from build123d import *

# Parameters (mm, degrees)
SKETCH1_R                      = 4.1275
BOSS_EXTRUDE1_DEPTH            = 22.225
F_7_0_201_DIAMETER_HOLE1_D     = 5.1054
F_7_0_201_DIAMETER_HOLE1_DEPTH = 1.27
F_10_32_TAPPED_HOLE1_D         = 4.0386


with BuildPart() as part:
    # Sketch1 → Boss-Extrude1 (new body)
    with BuildSketch(Plane.XY):
        Circle(SKETCH1_R)
    extrude(amount=BOSS_EXTRUDE1_DEPTH)

    # #7 (0.201) Diameter Hole1
    with Locations(Plane(origin=(0, 4.1275, 9.525), x_dir=(1, 0, 0), z_dir=(0, 1, 0))):
        with Locations((0, 0)):
            Hole(F_7_0_201_DIAMETER_HOLE1_D / 2, depth=F_7_0_201_DIAMETER_HOLE1_DEPTH)

    # #10-32 Tapped Hole1 (through all)
    with Locations(Plane(origin=(0, 4.1275, 9.525), x_dir=(1, 0, 0), z_dir=(0, 1, 0))):
        with Locations((0, 0)):
            Hole(F_10_32_TAPPED_HOLE1_D / 2)


solid = part.part
Part model, mm, in its own coordinate system. Give positions to 0.01 mm unless a question says otherwise; leave off trailing zeros. Loops run counter-clockwise (first coordinate to the right, second up) from the corner with the lowest first, then second, coordinate; pieces in that order, holes last.
(1) Band-saw the part on D-D (y = -1). Write the cut outline in (x, z) (3 decimals).
Return value:
outline: (-4.005, 0) - (4.005, 0) - (4.005, 22.225) - (-4.005, 22.225) - close; hole circle Ø4.039 at (0, 9.525)
(2) Pull direction X, two halves, no side cores. Call faces 1 (the cylindrical face through (2.026, 3.345, 11.078)), 2 (the flat face through (0, 0, 0)), 3 (the cylindrical face through (1.905, -3.662, 10.957)), 4 (the cylindrical face through (2.017, -0.686, 9.436)): pulls with the +X half, pulls with the -X half, needs draft (parallel to the pull), parting line crosses it, or undercut.
Return value:
face 1: undercut
face 2: needs draft
face 3: parting line crosses it
face 4: undercut
(3) Drill centre lines: line 1 along Z through (x, y) = (0, 3.65) (3 decimals); line 2 along Z through (x, y) = (-1, -3) (3 decimals); line 3 along Y through (x, z) = (-2.5, 18). Where is each one in solid material? Low to high.
Return value:
line 1: z = 0 to 6.972, 12.078 to 22.225
line 2: z = 0 to 7.771, 11.279 to 22.225
line 3: y = -3.28 to 3.28
(4) Pin check, flat tip, straight feed: pin 1 (2 mm diameter, centred on y = 2, z = 14, fed in from -X). Stop position of the tip, or through.
Return value:
pin 1: stops at x = -4
(5) Band-saw the part on C-C (y = 3.5). Write the cut outline in (x, z) (3 decimals), and give its area (3 significant figures).
Return value:
outline: (-2.188, 0) - (2.188, 0) - (2.188, 8.21) arc R2.553 cw to (-2.188, 8.21) - close; (-2.188, 10.84) arc R2.553 cw to (2.188, 10.84) - (2.188, 22.225) - (-2.188, 22.225) - close
area: 78.1 mm2
(6) Band-saw the part on A-A (x = 0). Write the cut outline in (y, z) (1 decimal), and give its area (3 significant figures).
Return value:
outline: (-4.1, 0) - (4.1, 0) - (4.1, 7) - (2.9, 7) - (2.9, 7.5) - (-4.1, 7.5) - close; (-4.1, 11.5) - (2.9, 11.5) - (2.9, 12.1) - (4.1, 12.1) - (4.1, 22.2) - (-4.1, 22.2) - close
area: 149 mm2
